The listing builds one solid part. Answer for the finished solid, in the listing's coordinates (mm). A direction names the side the tool comes from. Coordinates: 2 decimals unless noted, no trailing zeros. Order: outer loops, then holes, each group sorted by start corner. A loop starts at its lowest first (then second) coordinate and runs counter-clockwise, first axis right, second up.
from build123d import *

# Parameters (mm, degrees)
SZKIC1_R                    = 11.1
DODANIE_WYCI_GNI_CIE1_DEPTH = 15
DODANIE_WYCI_GNI_CIE2_START = -5
SZKIC2_R                    = 11.1
SZKIC2_R_2                  = 4.25
DODANIE_WYCI_GNI_CIE2_DEPTH = 5
SZKIC3_R                    = 2.2
WYTNIJ_WYCI_GNI_CIE1_DEPTH  = 71.662295462


with BuildPart() as part:
    # Szkic1 → Dodanie-wyciągnięcie1 (new body)
    with BuildSketch(Plane.XY):
        Polygon((25.2, -56), (25.2, -28.9), (15.2, 8), (10.2, 8), (10.2, -8), (-10.2, -8), (-10.2, 8), (-15.2, 8), (-15.2, -56), align=None)
        with Locations((9.2, -40)):
            Circle(SZKIC1_R, mode=Mode.SUBTRACT)
    extrude(amount=DODANIE_WYCI_GNI_CIE1_DEPTH)

    # Szkic2 → Dodanie-wyciągnięcie2 (add)
    with BuildSketch(Plane.XY.offset(15).offset(DODANIE_WYCI_GNI_CIE2_START)):
        with Locations((9.2, -40)):
            Circle(SZKIC2_R)
        with Locations((9.2, -40)):
            Circle(SZKIC2_R_2, mode=Mode.SUBTRACT)
    extrude(amount=DODANIE_WYCI_GNI_CIE2_DEPTH)

    # Szkic3 → Wytnij-wyciągnięcie1 (cut, through all)
    with BuildSketch(Plane.ZY.offset(15.2)):
        with Locations(Location((7.5, 0, 0), (0, 0, 270))):
            Circle(SZKIC3_R)
    extrude(amount=-WYTNIJ_WYCI_GNI_CIE1_DEPTH, mode=Mode.SUBTRACT)


solid = part.part
(1) Find section D-D on z = 7.5. Determine the outline of the cut face in (x, y), then the cut area to 3 significant figures.
(2) Find section A-A on x = 9.2. Determine the outline of the cut face in (y, z).
(3) Find section B-B on y = -40. Determine the outline of the cut face in (x, z), then the cut area to 4 significant figures.
(4) Find the intervals of material crossed by probe 1 along Z at (x, y) = (15, 0); probe 2 along Y at (x, z) = (9.2, 6.5); probe 3 along Y at (x, z) = (9.2, 13.1), in increasing order.
(5) Find section C-C on z = 11.75. Determine the outline of the cut face in (x, y), then the cut area to 3 significant figures.
(6) Given pin 1 Ø20 at (x, y) = (9.2, -40) entering from +Z; pin 2 Ø3 at (x, z) = (-7.5, 2.5) entering from +Y; pin 3 Ø7.5 at (y, z) = (-1, 7) entering from +X, each flat-ended and moving along its own axis, determine where each tip first touches the part or whether it passes through.
(7) The mould has two halves that part along X. Classify faces 1 (the flat face through (-15.2, -24, 7)), 2 (the cylindrical face through (8.647, -35.786, 12.465)), 3 (the flat face through (25.2, -43, 7)): pulls with the +X half, pulls with the -X half, needs draft (parallel to the pull), parting line crosses it, or undercut.
(8) A tool of negligible diameter and unlimited length cuts with its end or side. For faces 4 (the flat face through (10.2, 2, 9)), 5 (the flat face through (5, -56, 7)), 6 (the flat face through (14, -40, 10)), from which of +Z, -Z, +X, -X, +Y, -Y can it reach the whole face along a straight path? Write none if from no direction.
Resolved:
1. outline: (-15.2, -56) - (25.2, -56) - (25.2, -28.9) - (17.96, -2.2) - (10.2, -2.2) - (10.2, -8) - (-10.2, -8) - (-10.2, -2.2) - (-15.2, -2.2) - close; (-15.2, 2.2) - (-10.2, 2.2) - (-10.2, 8) - (-15.2, 8) - close; (10.2, 2.2) - (16.77, 2.2) - (15.2, 8) - (10.2, 8) - close; hole circle Ø22.2 at (9.2, -40)
1. area: 1,630 mm2
2. outline: (-56, 0) - (-51.1, 0) - (-51.1, 10) - (-44.25, 10) - (-44.25, 15) - (-56, 15) - close; (-35.75, 10) - (-28.9, 10) - (-28.9, 0) - (-8, 0) - (-8, 15) - (-35.75, 15) - close
3. outline: (-15.2, 0) - (-1.9, 0) - (-1.9, 10) - (4.95, 10) - (4.95, 15) - (-15.2, 15) - close; (13.45, 10) - (20.3, 10) - (20.3, 0) - (25.2, 0) - (25.2, 15) - (13.45, 15) - close
3. area: 341.5 mm2
4. probe 1: z = 0 to 5.3, 9.7 to 15
4. probe 2: y = -56 to -51.1, -28.9 to -8
4. probe 3: y = -56 to -44.25, -35.75 to -8
5. outline: (-15.2, -56) - (25.2, -56) - (25.2, -28.9) - (15.2, 8) - (10.2, 8) - (10.2, -8) - (-10.2, -8) - (-10.2, 8) - (-15.2, 8) - close; hole circle Ø8.5 at (9.2, -40)
5. area: 2,020 mm2
6. pin 1: stops at z = 15
6. pin 2: stops at y = -8
6. pin 3: stops at x = 18.66
7. face 1: pulls with the -X half
7. face 2: undercut
7. face 3: pulls with the +X half
8. face 4: +Z, -Z, +Y
8. face 5: +Z, -Z, +X, -X, -Y
8. face 6: -Z
